Geometry: final body of the model. Coordinates: model frame, mm. A direction names the side the tool comes from. Give positions to 0.01 mm unless a question says otherwise; leave off trailing zeros. Write each loop counter-clockwise with the first axis right and the second up, starting at its lowest first coordinate (ties: lowest second). Pieces come first, ordered by that corner, then holes.
Q1. Cut plane A-A on z = 10.75. Return the cut outline in (x, y).
Q2. Line query: L1, parallel to X at y = 7.5, z = 12.5; L2, parallel to X at y = 6.5, z = 15.75; L3, parallel to X at y = -18.5, z = 16.5. Output: solid intervals per line, ascending.
Q3. Reachability of faces 4 (the face through (41, -12.7, 18)), 5 (the face through (-38.853, -0.32, 10.558)) from +Z, -Z, +X, -X, +Y, -Y: full face, straight path, thin tool, end or side. Return the list, or none.
Q4. Cut plane B-B on x = -10. Return the cut outline in (y, z), plus the area to 3 significant figures.
Q5. Draft query along Z for faces 1 (the face through (39, -5, 14.357)), 2 (the face through (17.109, -0.32, 7.513)), 3 (the face through (46.101, 0, 10)). Return one class per face: pulls with the +Z half, pulls with the -Z half, needs draft (parallel to the pull), parting line crosses it, or undercut.
Q6. Pin query (flat end, axial travel): pin 1 (2 mm diameter, centred on x = 36, y = -16, fed in from +Z); pin 2 (3 mm diameter, centred on x = 20, y = 16.5, fed in from +Z); pin 3 (5.5 mm diameter, centred on x = 39, z = 17.5, fed in from -Y). Return the tip coordinate at first contact, or that it passes through.
Q7. Cut plane C-C on x = -28. Return the cut outline in (y, z), plus the area to 3 significant figures.
```python
from build123d import *

# Parameters (mm, degrees)
F1_DEPTH    = 22.86
F2_R        = 5.08
F3_R        = 0.762
F4_R        = 0.762
F5_W        = 14.2031247761
F5_H        = 10.16
F6_DEPTH    = 6.604
F7_T1_DEPTH = 67.1823585695


# Not quite as in the source:
# - a fillet or chamfer that OpenCascade refuses, or shapes differently, is made with other operations: its cross-section is extruded or revolved along the edge and cut away or added


with BuildPart() as f1:
    # F0 (on Front) → F1 (new body, symmetric)
    with BuildSketch(Plane.XZ):
        with BuildLine():
            Line((-35.941, 20.9608385392), (-46.101, 20.9608385392))
            Line((-46.101, 20.9608385392), (-46.101, 4.1968385392))
            Line((-46.101, 4.1968385392), (0, 4.1968385392))
            Line((0, 4.1968385392), (46.101, 4.1968385392))
            Line((46.101, 4.1968385392), (46.101, 20.9608385392))
            Line((46.101, 20.9608385392), (35.941, 20.9608385392))
            Line((35.941, 20.9608385392), (35.941, 15.8808385392))
            Line((35.941, 15.8808385392), (41.021, 15.8808385392))
            Line((41.021, 15.8808385392), (41.021, 14.3568385392))
            Line((41.021, 14.3568385392), (35.9785540412, 14.3568385392))
            Line((35.9785540412, 14.3568385392), (36.0038614542, 12.846416393))
            ThreePointArc((36.0038614542, 12.846416393), (35.4291085131, 10.2844081543), (33.7465347616, 8.2686768405))
            Line((33.7465347616, 8.2686768405), (0, 6.7368385392))
            Line((0, 6.7368385392), (-33.7465347616, 8.2686768405))
            ThreePointArc((-33.7465347616, 8.2686768405), (-38.9099642803, 10.6162670887), (-41.021, 15.8808385392))
            Line((-41.021, 15.8808385392), (-35.941, 15.8808385392))
            Line((-35.941, 15.8808385392), (-35.941, 20.9608385392))
        make_face()
    extrude(amount=F1_DEPTH, both=True)

    # F2
    f2_edges = [f1.edges().sort_by_distance(p)[0] for p in [
        (-46.101, 0, 20.960839),
        (46.101, 0, 20.960839),
    ]]
    fillet(f2_edges, radius=F2_R)

    # F3
    f3_edges = [f1.edges().sort_by_distance(p)[0] for p in [
        (35.978554, 0, 14.356839),
    ]]
    fillet(f3_edges, radius=F3_R)

    # F4
    f4_edges = [f1.edges().sort_by_distance(p)[0] for p in [
        (35.941, 0, 15.880839),
    ]]
    fillet(f4_edges, radius=F4_R)

    # F5 (on face) → F6 (cut, through all)
    with BuildSketch(Plane.XY.offset(20.9608385392)):
        with Locations((43.0425623881, -17.78)):
            Rectangle(F5_W, F5_H)
    extrude(amount=-F6_DEPTH, mode=Mode.SUBTRACT)

    # F7: fillet of radius 4.2924717139 on 1 edges, made by hand

    # F7_s2 → F7_t1 (cut)
    with BuildSketch(Plane.XZ.offset(-33.5911792847)):
        with BuildLine():
            add(Edge.make_bspline(
                [(-35.941, 16.6683668253), (-35.941, 20.9608385392), (-40.2334717139, 20.9608385392)],
                knots=[0, 0, 0, 1, 1, 1], degree=2, weights=[1, 1, 1]))
            Line((-40.2334717139, 20.9608385392), (-35.941, 20.9608385392))
            Line((-35.941, 20.9608385392), (-35.941, 16.6683668253))
        make_face()
    extrude(amount=F7_T1_DEPTH, mode=Mode.SUBTRACT)


solid = f1.part
```
Data:
1. outline: (-46.1, -22.86) - (-39.03, -22.86) - (-39.03, 22.86) - (-46.1, 22.86) - close; (35.63, -22.86) - (46.1, -22.86) - (46.1, 22.86) - (35.63, 22.86) - close
2. L1: x = -46.1 to -40.23, 36 to 46.1
2. L2: x = -46.1 to -41.02, 41.02 to 46.1
2. L3: x = -46.06 to -35.94
3. face 4: +Z, +X, -Y
3. face 5: +Y, -Y
4. outline: (-22.86, 4.2) - (22.86, 4.2) - (22.86, 7.19) - (-22.86, 7.19) - close
4. area: 137 mm2
5. face 1: undercut
5. face 2: pulls with the +Z half
5. face 3: needs draft
6. pin 1: stops at z = 14.36
6. pin 2: stops at z = 7.71
6. pin 3: stops at y = -12.7
7. outline: (-22.86, 4.2) - (22.86, 4.2) - (22.86, 8.01) - (-22.86, 8.01) - close
7. area: 174 mm2
